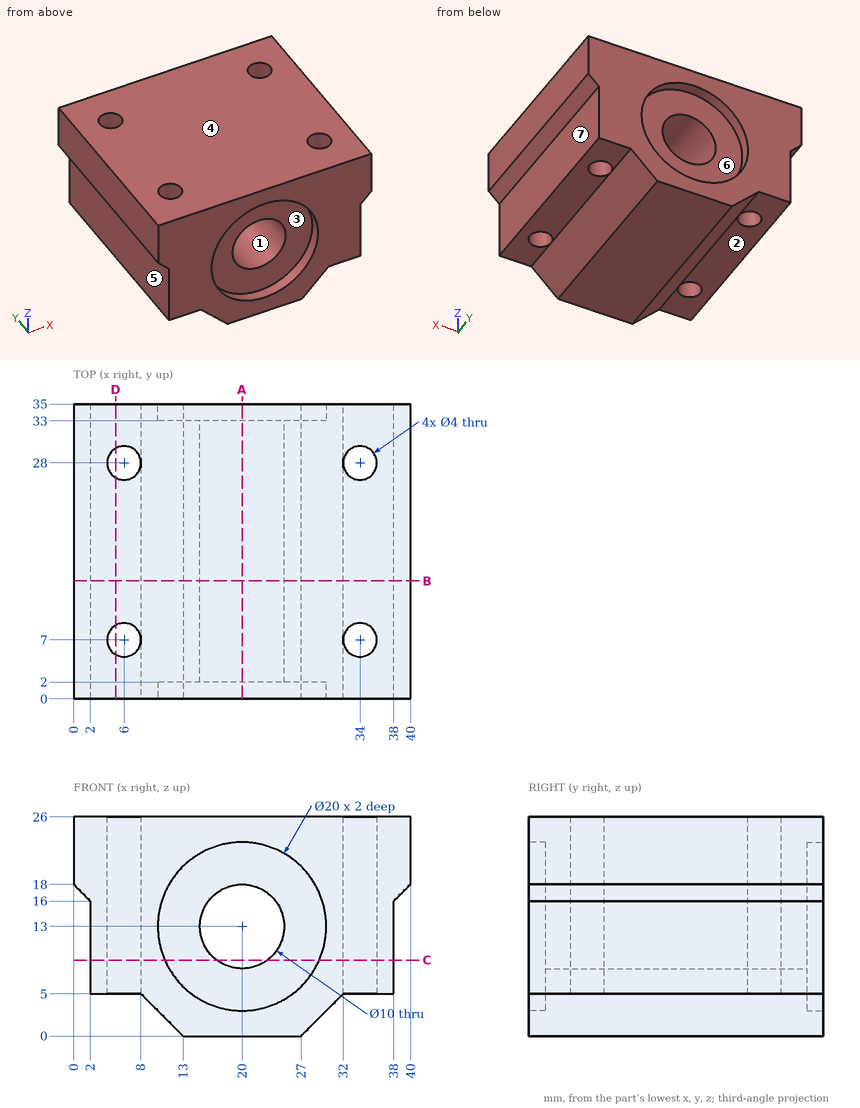
Source: three-view drawing plus pictorial views. Frame: mm from the lowest corner of the part. A direction names the side the tool comes from. Give positions to 0.01 mm unless a question says otherwise; leave off trailing zeros. Order: outer loops, then holes, each group sorted by start corner. A loop starts at its lowest first (then second) coordinate and runs counter-clockwise, first axis right, second up. Notation, with made-up numbers: M 69,-16 L 124,-16 A7 cw 124,-12 Z; hole C -6,89 d11. An arc over 180 degrees is marked long. One line per question, with ' | ' between items.
1) Draft query along Z for the marked faces 1, 2, 3 and 4. Return one class per face: pulls with the +Z half, pulls with the -Z half, needs draft (parallel to the pull), parting line crosses it, or undercut.
Filled in:
face 1: undercut | face 2: pulls with the -Z half | face 3: undercut | face 4: pulls with the +Z half
2) Section B-B on y = 14. Output: boundary loops of the cut face in (x, z).
Filled in:
outline: M 0,18 L 2,16 L 2,5 L 8,5 L 13,0 L 27,0 L 32,5 L 38,5 L 38,16 L 40,18 L 40,26 L 0,26 Z; hole C 20,13 d10
3) Access query for the marked faces 5, 6 and 7. Directions: +Z, -Z, +X, -X, +Y, -Y. A direction counts if a zero-diameter tool reaches every point of the face in a straight line with its end or side. Return the directions, or none.
Filled in:
face 5: -Z, -X, +Y, -Y | face 6: +Y | face 7: -Z, +X, +Y, -Y
4) Section A-A on x = 20. Output: boundary loops of the cut face in (y, z), and give its area (3 significant figures).
Filled in:
outline: M 0,0 L 35,0 L 35,3 L 33,3 L 33,8 L 2,8 L 2,3 L 0,3 Z; M 0,23 L 2,23 L 2,18 L 33,18 L 33,23 L 35,23 L 35,26 L 0,26 Z | area: 520 mm2
5) Contact query for flat-ended pins moving along their axis: P1, Ø12, axis at y = 22.5, z = 11.5, coming from the -X side; P2, Ø12, axis at x = 20, z = 13, coming from the +Y side; P3, Ø8, axis at x = 20, z = 13, coming from the -Y side; P4, Ø3, axis at y = 6.5, z = 6.5, coming from the +X side. Output: stop coordinate, or through.
Filled in:
P1: stops at x = 0.5 | P2: stops at y = 33 | P3: passes through | P4: stops at x = 38
6) Section D-D on x = 5. Output: boundary loops of the cut face in (y, z), and give its area (3 significant figures).
Filled in:
outline: M 0,5 L 5.27,5 L 5.27,26 L 0,26 Z; M 8.73,5 L 26.27,5 L 26.27,26 L 8.73,26 Z; M 29.73,5 L 35,5 L 35,26 L 29.73,26 Z | area: 590 mm2
7) Section C-C on z = 9. Output: boundary loops of the cut face in (x, y).
Filled in:
outline: M 2,0 L 10.83,0 L 10.83,2 L 17,2 L 17,33 L 10.83,33 L 10.83,35 L 2,35 Z; M 23,2 L 29.17,2 L 29.17,0 L 38,0 L 38,35 L 29.17,35 L 29.17,33 L 23,33 Z; hole C 6,7 d4; hole C 6,28 d4; hole C 34,7 d4; hole C 34,28 d4
8) Ray query, L1, parallel to Y at x = 32.5, z = 15.5; L2, parallel to Y at x = 34, z = 12; L3, parallel to Z at x = 31, y = 8. Return the intervals inside material, ascending.
Filled in:
L1: y = 0 to 5.68, 8.32 to 26.68, 29.32 to 35 | L2: y = 0 to 5, 9 to 26, 30 to 35 | L3: z = 4 to 26
